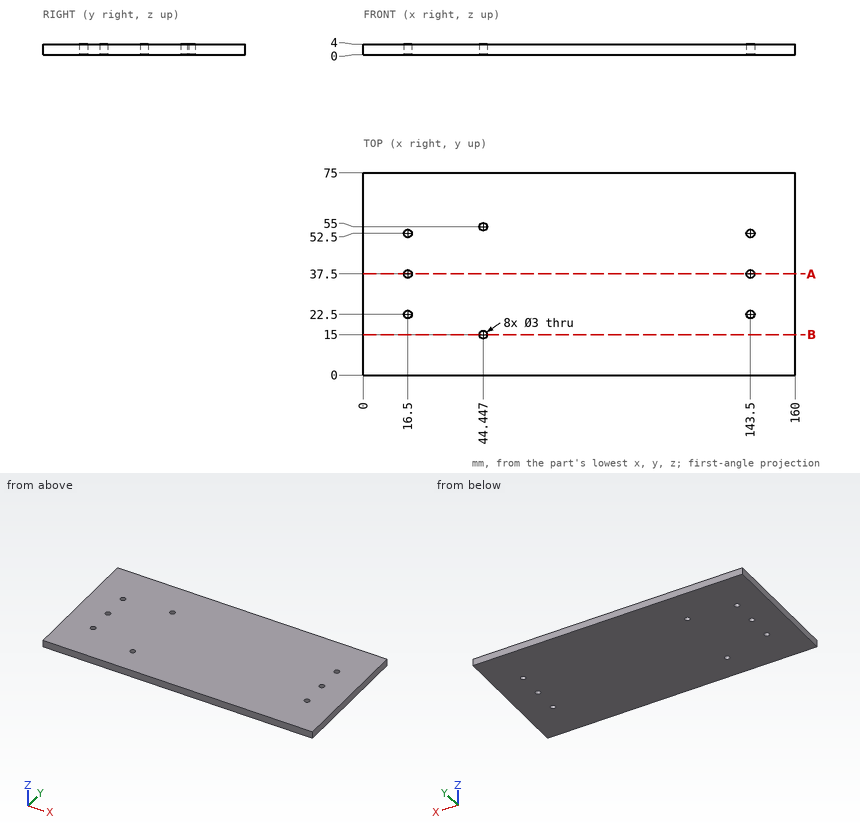
Input: dimensioned drawing with shaded views. Units: mm. Origin: part minimum x, y, z. Coordinates: 2 decimals unless noted, no trailing zeros. Loops run counter-clockwise (first coordinate to the right, second up) from the corner with the lowest first, then second, coordinate; pieces in that order, holes last.
Q1. Line query: line 1 along Y through (x, z) = (16.5, 1.3); line 2 along X through (y, z) = (36.5, 1.3); line 3 along Y through (x, z) = (44, 0.85). Output: solid intervals per line, ascending.
Results are:
line 1: y = 0 to 21, 24 to 36, 39 to 51, 54 to 75
line 2: x = 0 to 15.38, 17.62 to 142.38, 144.62 to 160
line 3: y = 0 to 13.57, 16.43 to 53.57, 56.43 to 75
Q2. Section A-A, the plane y = 37.5. Return the cut outline in (x, z).
Results are:
outline: (0, 0) - (15, 0) - (15, 4) - (0, 4) - close; (18, 0) - (142, 0) - (142, 4) - (18, 4) - close; (145, 0) - (160, 0) - (160, 4) - (145, 4) - close
Q3. Contact query for flat-ended pins moving along their axis: pin 1 (2.5 mm diameter, centred on x = 16.5, y = 37.5, fed in from -Z); pin 2 (5 mm diameter, centred on x = 143.5, y = 37.5, fed in from +Z). Output: stop coordinate, or through.
Results are:
pin 1: passes through
pin 2: stops at z = 4
Q4. Section B-B, the plane y = 15. Return the cut outline in (x, z), and give its area (3 significant figures).
Results are:
outline: (0, 0) - (42.95, 0) - (42.95, 4) - (0, 4) - close; (45.95, 0) - (160, 0) - (160, 4) - (45.95, 4) - close
area: 628 mm2
